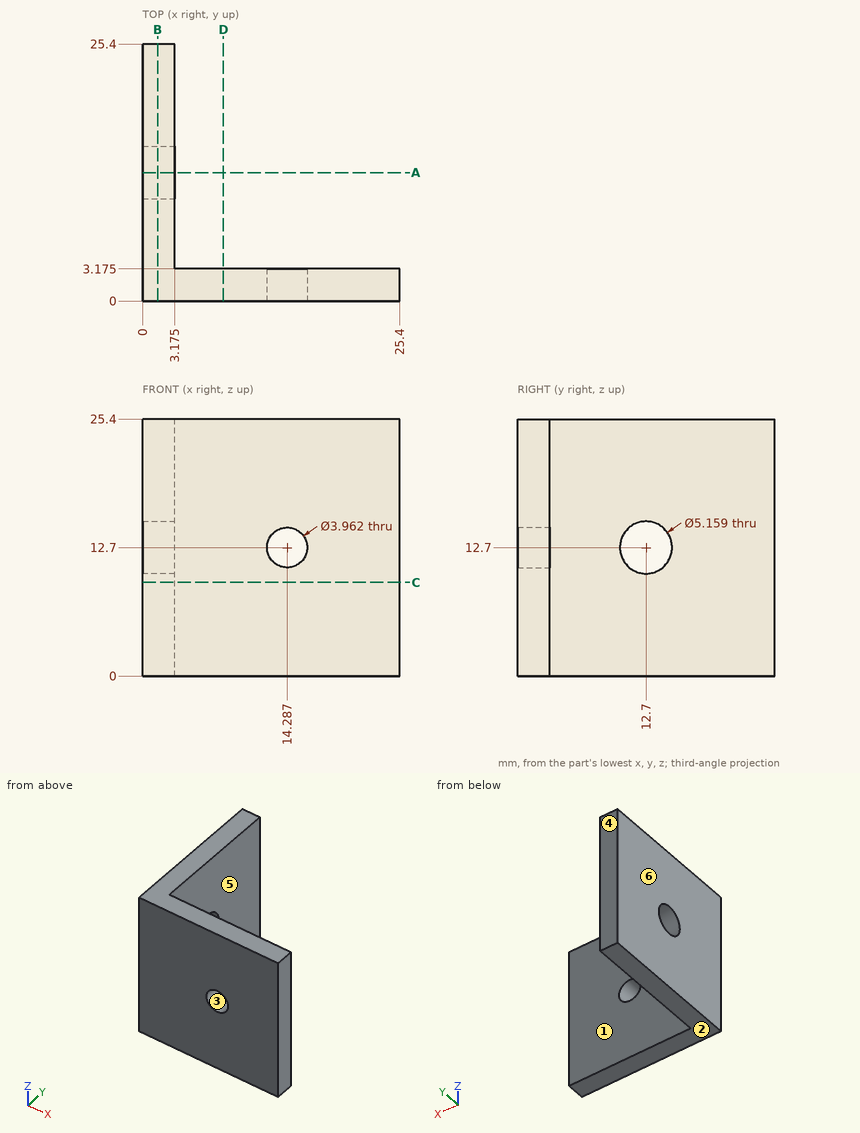
Answer from the drawing. Dimensions are ordinates in mm from the lowest x, y and z of the part. A direction names the side the tool comes from. Give positions to 0.01 mm unless a question says otherwise; leave off trailing zeros. Order: outer loops, then holes, each group sorted by start corner. A loop starts at its lowest first (then second) coordinate and runs counter-clockwise, first axis right, second up.
Item 1: The part is cut by section C-C, the plane z = 9.25. Give the vertices of the cut face in (x, y) (1 decimal), and give its area (3 significant figures).
From the geometry:
outline: (0, 0) - (25.4, 0) - (25.4, 3.2) - (3.2, 3.2) - (3.2, 25.4) - (0, 25.4) - close
area: 151 mm2
Item 2: The part is cut by section D-D, the plane x = 8. Give the vertices of the cut face in (y, z) (1 decimal).
From the geometry:
outline: (0, 0) - (3.2, 0) - (3.2, 25.4) - (0, 25.4) - close
Item 3: Find the intervals of material crossed by probe 1 along X at (y, z) = (1.75, 12.7); probe 2 along Y at (x, z) = (1.6, 12.7); probe 3 along X at (y, z) = (13.25, 6.5) (1 decimal), in increasing order.
From the geometry:
probe 1: x = 0 to 12.31, 16.27 to 25.4
probe 2: y = 0 to 10.12, 15.28 to 25.4
probe 3: x = 0 to 3.2
Item 4: The part is cut by section B-B, the plane x = 1.5. Give the vertices of the cut face in (y, z).
From the geometry:
outline: (0, 0) - (25.4, 0) - (25.4, 25.4) - (0, 25.4) - close; hole circle Ø5.16 at (12.7, 12.7)
Item 5: Which of the six approach directions +Z, -Z, +X, -X, +Y, -Y give full straight-line access (tool end or side, diameter ignored) to the marked faces 1 and 2?
From the geometry:
face 1: +Z, -Z, +X, +Y
face 2: -Z, +X, -X, +Y, -Y
Item 6: Given pin 1 Ø5 at (y, z) = (14.5, 17.5) entering from +X (1 decimal); pin 2 Ø6.5 at (x, z) = (11.5, 7.5) entering from +Y (1 decimal), each flat-ended and moving along its own axis, determine where each tip first touches the part or whether it passes through.
From the geometry:
pin 1: stops at x = 3.2
pin 2: stops at y = 3.2
Item 7: For a pull along X with two mould halves and no side action, classify the marked faces 3, 4, 5 and 6 as pulls with the +X half, pulls with the -X half, needs draft (parallel to the pull), parting line crosses it, or undercut.
From the geometry:
face 3: undercut
face 4: needs draft
face 5: pulls with the +X half
face 6: pulls with the -X half
Item 8: The part is cut by section A-A, the plane y = 12.7. Give the vertices of the cut face in (x, z) (1 decimal).
From the geometry:
outline: (0, 0) - (3.2, 0) - (3.2, 10.1) - (0, 10.1) - close; (0, 15.3) - (3.2, 15.3) - (3.2, 25.4) - (0, 25.4) - close
